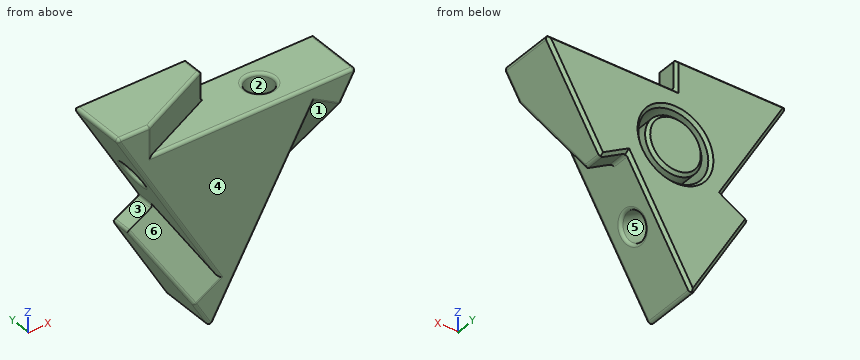
```python
from build123d import *

# Parameters (mm, degrees)
SKETCH1_R           = 7.2
BOSS_EXTRUDE1_DEPTH = 12
SKETCH2_R           = 7.2
BOSS_EXTRUDE2_DEPTH = 2
SKETCH3_R           = 2.7999999999999985
CUT_EXTRUDE1_DEPTH  = 9.1
CUT_EXTRUDE3_DEPTH  = 50.58533021602103
SKETCH8_R           = 5.8
BOSS_EXTRUDE3_DEPTH = 10
CIRPATTERN2_COUNT   = 3
CHAMFER2_SIZE       = 0.6
FILLET3_R           = 0.6


with BuildPart() as part:
    # Sketch1 → Boss-Extrude1 (new body)
    with BuildSketch(Plane(origin=(0, 0, 0), x_dir=(1, 0, 0), z_dir=(0, 1, 0))):
        Polygon((-23.110809387790948, -17.47636535456504), (-9.76561885940777, 5.638182677282097), (-15.134976362871324, 8.738182677282033), (-3.579571668975892, 28.752730709129278), (9.765618859407624, 5.638182677282344), (15.13497636287113, 8.738182677282364), (26.690381056766807, -11.276365354564588), (0, -11.27636535456458), (0, -17.476365354564578), align=None)
        with Locations(Location((0, 0, 0), (0, 0, 270))):
            Circle(SKETCH1_R, mode=Mode.SUBTRACT)
    extrude(amount=BOSS_EXTRUDE1_DEPTH)

    # Sketch2 → Boss-Extrude2 (add)
    with BuildSketch(Plane.XZ):
        with Locations(Location((0, 0, 0), (0, 0, 270))):
            Circle(SKETCH2_R)
    extrude(amount=-BOSS_EXTRUDE2_DEPTH)

    # Sketch3 → Cut-Extrude1 (cut)
    with BuildSketch(Plane.XY.offset(11.27636535456458)):
        with Locations((10.899999999999999, 6)):
            Circle(SKETCH3_R)
    cut_extrude1 = extrude(amount=-CUT_EXTRUDE1_DEPTH, mode=Mode.SUBTRACT)

    # Sketch7 → Cut-Extrude3 (cut, through all)
    with BuildSketch(Plane.XY.offset(11.27636535456458)):
        with BuildLine():
            Line((13.43570957044416, 0.5621532777800846), (-23.41303642284339, -16.620699172297943))
            ThreePointArc((-23.41303642284339, -16.620699172297943), (-31.38659271550747, -13.718562020522187), (-28.484455563731718, -5.7450057278581115))
            Line((-28.484455563731718, -5.7450057278581115), (8.364290429555835, 11.437846722219916))
            ThreePointArc((8.364290429555835, 11.437846722219916), (16.337846722219915, 8.535709570444162), (13.43570957044416, 0.5621532777800846))
        make_face()
    cut_extrude3 = extrude(amount=CUT_EXTRUDE3_DEPTH, mode=Mode.SUBTRACT)

    # Sketch8 → Boss-Extrude3 (add)
    with BuildSketch(Plane(origin=(0, 2, 0), x_dir=(1, 0, 0), z_dir=(0, 1, 0))):
        with Locations(Location((0, 0, 0), (0, 0, 90))):
            Circle(SKETCH8_R)
    extrude(amount=BOSS_EXTRUDE3_DEPTH)

    # CirPattern2: Cut-Extrude1, Cut-Extrude3 ×3 about axis
    cirpattern2_axis = Axis((-8e-16, 0, -3.09e-15), (0, 1, 0))
    add([cut_extrude1.rotate(cirpattern2_axis, i * 360 / CIRPATTERN2_COUNT) for i in range(1, CIRPATTERN2_COUNT)], mode=Mode.SUBTRACT)
    add([cut_extrude3.rotate(cirpattern2_axis, i * 360 / CIRPATTERN2_COUNT) for i in range(1, CIRPATTERN2_COUNT)], mode=Mode.SUBTRACT)

    # Chamfer2
    chamfer2_edges = [part.edges().sort_by_distance(p)[0] for p in [
        (13.345190528383403, 12, 11.276365354564584),
        (20.91267870981897, 12, 1.2690913386411111),
        (12.450297611139376, 12, -7.188182677282353),
        (2.2e-15, 12, -7.2),
        (3.0930235952158665, 12, -17.19545669320581),
        (-9.357274015923608, 12, -18.745456693205654),
        (-12.450297611139547, 12, -7.1881826772820645),
        (-16.43821412359936, 12, 5.919091338641472),
        (-11.555404693895474, 12, 17.47636535456481),
        (-1.07e-15, 12, 5.8),
        (0, 12, 14.37636535456458),
    ]]
    chamfer(chamfer2_edges, length=CHAMFER2_SIZE)

    # Fillet3
    fillet3_edges = [part.edges().sort_by_distance(p)[0] for p in [
        (-5.316211260430414, 0, -25.744782702294316),
        (-11.093913607378132, 3.76875701994284, -15.737508686370697),
        (-4.3681721001530995, 0, -21.186834695459314),
        (7.134086350709061, 0, -10.196130684117296),
        (24.953741465312213, 0, 8.268417347729613),
        (5.263065017397029, 0, 11.276365354564584),
        (-19.63753020488185, 0, 17.47636535456497),
        (-23.110809387790948, 5.700000000000001, 17.47636535456504),
        (-9.76561885940777, 9.468757019942823, -5.638182677282097),
        (-15.134976362871324, 9.468757019942839, -8.738182677282033),
        (-3.579571668975892, 5.700000000000001, -28.752730709129278),
        (9.765618859407624, 9.46875701994278, -5.638182677282344),
        (15.13497636287113, 9.468757019942785, -8.738182677282364),
        (26.690381056766807, 5.7, 11.276365354564588),
        (0, 9.468757019942768, 11.27636535456458),
        (0, 9.468757019942766, 17.476365354564578),
        (8.099999999999996, 6, 11.27636535456458),
        (-8.082125510986373, 3.7687570199427665, 17.476365354564738),
        (-16.164251021972746, 0, 14.376365354564811),
        (-13.815618859407646, 6, 1.3766230933716486),
        (5.715618859407651, 6, -12.652988447936243),
        (19.176039118364372, 3.7687570199427864, -1.7388566681938666),
        (20.532423122125817, 0, 6.810469340894656),
        (-12.397151368106105, 0, -1.0802346704471155),
    ]]
    fillet(fillet3_edges, radius=FILLET3_R)


solid = part.part
```
For this review, take the finished solid that the model builds, in its own axes (mm). Face numbers are marked on the shaded views. A direction names the side the tool comes from. Coordinates: 2 decimals unless noted, no trailing zeros. Order: outer loops, then holes, each group sorted by start corner. A loop starts at its lowest first (then second) coordinate and runs counter-clockwise, first axis right, second up. Notation, with made-up numbers: (-8, 46) - (24, 46) arc R29 ccw to (24, 68) - close; hole circle Ø6 at (31.25, 5.25). An arc over 180 degrees is marked (long way). Answer as a JSON object with one key per item and string values. Group by question number.
1. We need section A-A on y = 10.5. State the section outline as (x, z) points.
2. We need section B-B on y = 5.25. Give the number of separate pieces and of enclosed holes in the cut face, then the cut area to 3 significant figures.
3. For the marked faces 1, 2 and 3, list the 3-axis set-ups (+Z, -Z, +X, -X, +Y, -Y) from which the entire face can be reached by the end or side of a thin tool; tool diameter is ignored.
4. For probe 1 along X at (y, z) = (3.75, -5); probe 2 along X at (y, z) = (10.25, -4.5); probe 3 along Y at (x, z) = (10.9, 9.25), list the stretches that pass through material, from the lowest coordinate up.
5. Clearance check with flat-ended pins moving along their axes: P1, Ø4, axis at x = -16, z = 6.5, coming from the -Y side; P2, Ø5, axis at x = 19, y = 2, coming from the +Z side; P3, Ø1, axis at y = 5, z = -19, coming from the +X side; P4, Ø4, axis at y = 2.5, z = -7.5, coming from the +X side. State where each tip first meets the part, or that it passes through.
6. The part is to be moulded in two halves that separate along X. For the marked faces 4, 5 and 6, say which applies: pulls with the +X half, pulls with the -X half, needs draft (parallel to the pull), parting line crosses it, or undercut.
Final values:
{
 "1": {"outline": "(-22.59, 16.58) - (-10.07, -5.12) arc R0.6 cw to (-10.29, -5.94) - (-14.62, -8.44) arc R0.6 ccw to (-14.83, -9.26) - (-4.1, -27.85) arc R0.6 ccw to (-3.06, -27.85) - (9.47, -6.16) arc R0.6 cw to (10.29, -5.94) - (14.62, -8.44) arc R0.6 ccw to (15.43, -8.22) - (26.17, 10.38) arc R0.6 ccw to (25.65, 11.28) - (0.6, 11.28) arc R0.6 cw to (0, 11.88) - (0, 16.88) arc R0.6 ccw to (-0.6, 17.48) - (-22.07, 17.48) arc R0.6 ccw to start; circle Ø11.6 at (0, 0); hole circle Ø14.4 at (0, 0)"},
 "2": {"separate pieces": "2", "enclosed holes": "1", "area": "760 mm²"},
 "3": {"face 1": "-Z, -Y", "face 2": "+Z", "face 3": "-X, +Y, -Y"},
 "4": {"probe 1": "-10.13 to -5.18, -2.94 to 2.94, 5.18 to 10.13", "probe 2": "-10.42 to -5.62, -3.66 to 3.66, 5.62 to 17.58", "probe 3": "0 to 3.2, 8.8 to 12"},
 "5": {"P1": "y = 0", "P2": "z = 11.28", "P3": "x = 2.34", "P4": "x = 9.85"},
 "6": {"face 4": "needs draft", "face 5": "undercut", "face 6": "pulls with the -X half"}
}
